The model under review builds one solid part; all positions refer to its coordinate system, in mm. A direction names the side the tool comes from. Round coordinates to 2 decimals unless told otherwise and drop trailing zeros. Loops run counter-clockwise (first coordinate to the right, second up) from the corner with the lowest first, then second, coordinate; pieces in that order, holes last. Notation, with made-up numbers: (2, -31.5) -> (40, -31.5) arc R25 cw to (40, 6.5) -> close; hole circle Ø2 at (87, 20.5). An arc over 180 degrees is marked (long way). Use a Markdown table: item, result. Add a question column.
1) Consider section C-C on y = 2.75. Give the boundary of the cut face in (x, z).
2) Insertion check: pin 1 (3 mm diameter, centred on x = -2, z = -1, fed in from -Y); pin 2 (1.5 mm diameter, centred on x = -5, z = -2, fed in from +Y); pin 3 (0.6 mm diameter, centred on x = 5, z = -26, fed in from -Y). Each pin has a flat end and moves straight along its axis. Give the tip position at first contact, or say it passes through.
3) Consider section A-A on x = 0. Give the boundary of the cut face in (y, z).
4) Mouldability with a two-part tool opening along Z and no side actions: class faces 5 (the cylindrical face through (-5, 0, -29)), 6 (the cylindrical face through (-1.19, -5.37, 0.29)), 7 (the flat face through (-5, 0, 21)) as released by +Z, released by -Z, zero draft, split by the parting line, or undercut.
5) Wall thickness on probe 1 along Y at (x, z) = (0, -8.5); probe 2 along Z at (x, y) = (2.25, 1.5); probe 3 along Z at (x, y) = (5.35, 0): over which ranges is each line inside the solid? List them lowest first.
6) For faces 1 (the flat face through (-5, -3.5, -27)), 2 (the flat face through (5, 3.5, -27)), 3 (the flat face through (3.75, 0, -28.7)), 4 (the flat face through (6, 0, -21)), list the 3-axis set-ups (+Z, -Z, +X, -X, +Y, -Y) from which the entire face can be reached by the end or side of a thin tool; tool diameter is ignored.
7) Consider section B-B on z = 17. Give the boundary of the cut face in (x, y), plus the area to 3 significant figures.
8) Consider section D-D on x = 6.25. Give the boundary of the cut face in (y, z), plus the area to 3 significant figures.
from build123d import *

# Parameters (mm, degrees)
SKETCH1_R                = 5.5
YOKE_DEPTH               = 21
SKETCH2_R                = 6.75
U_JOINT_BASE_DEPTH       = 3
U_JOINT_STANDUPS_DEPTH   = 9.5
STANDUP_ROUND_DEPTH      = 7.75
STANDUP_ROUND_DEPTH_BACK = 7.75
SKETCH5_R                = 1
BALL_HOLES_DEPTH         = 7.75
BALL_HOLES_DEPTH_BACK    = 7.75
KEYWAY_DEPTH             = 42


with BuildPart() as part:
    # Sketch1 → Yoke (new body, symmetric)
    with BuildSketch(Plane.XY):
        Circle(SKETCH1_R)
    extrude(amount=YOKE_DEPTH, both=True)

    # Sketch2 → U Joint Base (add)
    with BuildSketch(Plane(origin=(0, 0, -21), x_dir=(-1, 0, 0), z_dir=(0, 0, -1))):
        Circle(SKETCH2_R)
    extrude(amount=U_JOINT_BASE_DEPTH)

    # Sketch3 → U Joint Standups (add)
    with BuildSketch(Plane(origin=(0, 0, -24), x_dir=(-1, 0, 0), z_dir=(0, 0, -1))):
        with BuildLine():
            Line((-5.771698, 3.5), (-3.75, 3.5))
            Line((-3.75, 3.5), (-3.75, -3.5))
            Line((-3.75, -3.5), (-5.771698, -3.5))
            ThreePointArc((-5.771698, -3.5), (-6.75, 0), (-5.771698, 3.5))
        make_face()
        with BuildLine():
            Line((3.75, -3.5), (3.75, 3.5))
            Line((3.75, 3.5), (5.771698, 3.5))
            ThreePointArc((5.771698, 3.5), (6.75, 0), (5.771698, -3.5))
            Line((5.771698, -3.5), (3.75, -3.5))
        make_face()
    extrude(amount=U_JOINT_STANDUPS_DEPTH)

    # Sketch4 → Standup Round (cut, two sides)
    with BuildSketch(Plane(origin=(0, 0, 0), x_dir=(0, 0, -1), z_dir=(1, 0, 0))) as standup_round_sk:
        with BuildLine():
            ThreePointArc((30, -3.5), (32.474874, -2.474874), (33.5, 0))
            Line((33.5, 0), (33.5, -3.5))
            Line((33.5, -3.5), (30, -3.5))
        make_face()
        with BuildLine():
            ThreePointArc((33.5, 0), (32.474874, 2.474874), (30, 3.5))
            Line((30, 3.5), (33.5, 3.5))
            Line((33.5, 3.5), (33.5, 0))
        make_face()
    extrude(amount=STANDUP_ROUND_DEPTH, mode=Mode.SUBTRACT)
    extrude(standup_round_sk.sketch, amount=-STANDUP_ROUND_DEPTH_BACK, mode=Mode.SUBTRACT)

    # Sketch5 → Ball Holes (cut, two sides)
    with BuildSketch(Plane(origin=(0, 0, 0), x_dir=(0, 0, -1), z_dir=(1, 0, 0))) as ball_holes_sk:
        with Locations((30, 0)):
            Circle(SKETCH5_R)
    extrude(amount=BALL_HOLES_DEPTH, mode=Mode.SUBTRACT)
    extrude(ball_holes_sk.sketch, amount=-BALL_HOLES_DEPTH_BACK, mode=Mode.SUBTRACT)

    # Sketch6 → Keyway (cut)
    with BuildSketch(Plane.XY.offset(21)):
        with BuildLine():
            Line((0.5, -4.472136), (0.5, -3.972136))
            Line((0.5, -3.972136), (-0.5, -3.972136))
            Line((-0.5, -3.972136), (-0.5, -4.472136))
            ThreePointArc((-0.5, -4.472136), (0, 4.5), (0.5, -4.472136))
        make_face()
    extrude(amount=-KEYWAY_DEPTH, mode=Mode.SUBTRACT)


solid = part.part
Result set:
| question | item | result |
|---|---|---|
| 1 | outline | (-6.16, -32.17) -> (-3.75, -32.17) -> (-3.75, -24) -> (3.75, -24) -> (3.75, -32.17) -> (6.16, -32.17) -> (6.16, -21) -> (4.76, -21) -> (4.76, 21) -> (3.56, 21) -> (3.56, -21) -> (-3.56, -21) -> (-3.56, 21) -> (-4.76, 21) -> (-4.76, -21) -> (-6.16, -21) -> close |
| 2 | pin 1 | y = -5.48 |
| 2 | pin 2 | y = 3.49 |
| 2 | pin 3 | y = -3.5 |
| 3 | outline | (-6.75, -24) -> (6.75, -24) -> (6.75, -21) -> (5.5, -21) -> (5.5, 21) -> (4.5, 21) -> (4.5, -21) -> (-3.97, -21) -> (-3.97, 21) -> (-5.5, 21) -> (-5.5, -21) -> (-6.75, -21) -> close |
| 4 | face 5 | undercut |
| 4 | face 6 | zero draft |
| 4 | face 7 | released by +Z |
| 5 | probe 1 | -5.5 to -3.97, 4.5 to 5.5 |
| 5 | probe 2 | -24 to -21 |
| 5 | probe 3 | -33.5 to -31, -29 to 21 |
| 6 | face 1 | -Z, +X, -X, -Y |
| 6 | face 2 | -Z, +X, -X, +Y |
| 6 | face 3 | -Z, +Y, -Y |
| 6 | face 4 | +Z |
| 7 | outline | circle Ø11 at (0, 0); hole (-0.5, -4.47) -> (-0.5, -3.97) -> (0.5, -3.97) -> (0.5, -4.47) arc R4.5 ccw (long way) to start |
| 7 | area | 31.9 mm2 |
| 8 | outline | (-2.55, -32.4) arc R3.5 ccw to (0, -33.5) arc R3.5 ccw to (2.55, -32.4) -> (2.55, -21) -> (-2.55, -21) -> close; hole circle Ø2 at (0, -30) |
| 8 | area | 58.9 mm2 |
